The listing builds one solid part. Answer for the finished solid, in the listing's coordinates (mm). Face numbers are marked on the shaded views. A direction names the side the tool comes from. Round coordinates to 2 decimals unless told otherwise and drop trailing zeros. Write each loop counter-clockwise with the first axis right and the second up, starting at its lowest first coordinate (ties: lowest second). Pieces come first, ordered by that corner, then holes. Notation, with made-up numbers: (-21, -11) -> (-14, -11) arc R19 cw to (-14, -5) -> close; hole circle Ø3 at (38.25, 50.5). An arc over 180 degrees is marked (long way). Write each question's results on one line, items separated by ' | '. Start each with the question number.
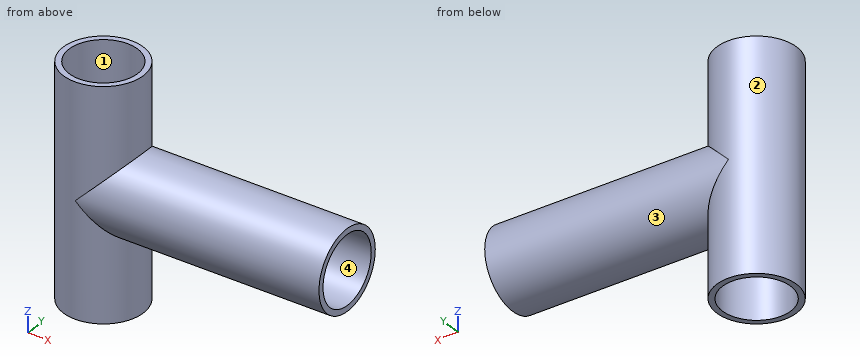
```python
from build123d import *

# Parameters (mm, degrees)
F0_R     = 17.5
F1_DEPTH = 100
F3_R     = 17.5
F4_DEPTH = 107.5
F5_R     = 15
F7_DEPTH = 95
F6_R     = 15
F8_DEPTH = 100


with BuildPart() as f1:
    # F0 (on Top) → F1 (new body)
    with BuildSketch(Plane.XY):
        Circle(F0_R)
    extrude(amount=F1_DEPTH)

    # F3 (on offset) → F4 (join)
    with BuildSketch(Plane.YZ.offset(107.5)):
        with Locations((0, 50)):
            Circle(F3_R)
    extrude(amount=-F4_DEPTH)

    # F5 (on face) → F7 (cut)
    with BuildSketch(Plane.YZ.offset(107.5)):
        with Locations((0, 50)):
            Circle(F5_R)
    extrude(amount=-F7_DEPTH, mode=Mode.SUBTRACT)

    # F6 (on face) → F8 (cut, through all)
    with BuildSketch(Plane.XY.offset(100)):
        Circle(F6_R)
    extrude(amount=-F8_DEPTH, mode=Mode.SUBTRACT)


solid = f1.part
```
Q1. The part is cut by section C-C, the plane z = 72. Write down the section's boundary in (x, y).
Q2. The part is cut by section D-D, the plane z = 50. Write down the section's boundary in (x, y).
Q3. Find the intervals of material crossed by line 1 (Z direction, x = 60, y = 0); line 2 (Y direction, x = 56, z = 50); line 3 (X direction, y = -10, z = 87), in increasing order.
Q4. Determine the mould class of the marked faces 3 and 4 for opening direction Y: pulls with the +Y half, pulls with the -Y half, needs draft (parallel to the pull), parting line crosses it, or undercut.
Q5. Each of these flat-tipped pins is pushed along its axis until it touches: pin 1 (1 mm diameter, centred on x = 89, y = 11.5, fed in from +Z); pin 2 (5.5 mm diameter, centred on y = 10.5, z = 49.5, fed in from +X); pin 3 (2 mm diameter, centred on y = 10, z = 18, fed in from -X). Where does it stop, or does it pass through?
Q6. The part is cut by section A-A, the plane y = 0. Write down the section's boundary in (x, z), then the cut area to 3 significant figures.
Q7. The part is cut by section B-B, the plane x = -8. Write down the section's boundary in (y, z).
Q8. For the marked faces 1 and 2, determine the directions among +Z, -Z, +X, -X, +Y, -Y from which every point of the face is accessible in a straight line to the end or side of a thin tool.
Answers follow:
1) outline: circle Ø35 at (0, 0); hole circle Ø30 at (0, 0)
2) outline: (0, -17.5) -> (107.5, -17.5) -> (107.5, -15) -> (12.5, -15) -> (12.5, -8.29) arc R15 cw (long way) to (12.5, 8.29) -> (12.5, 15) -> (107.5, 15) -> (107.5, 17.5) -> (0, 17.5) arc R17.5 ccw to start
3) line 1: 32.5 to 35, 65 to 67.5 | line 2: -17.5 to -15, 15 to 17.5 | line 3: -14.36 to -11.18, 11.18 to 14.36
4) face 3: parting line crosses it | face 4: undercut
5) pin 1: z = 63.61 | pin 2: x = 12.5 | pin 3: x = -15.01
6) outline: (-17.5, 0) -> (-15, 0) -> (-15, 100) -> (-17.5, 100) -> close; (15, 0) -> (17.5, 0) -> (17.5, 32.5) -> (107.5, 32.5) -> (107.5, 35) -> (15, 35) -> close; (15, 65) -> (107.5, 65) -> (107.5, 67.5) -> (17.5, 67.5) -> (17.5, 100) -> (15, 100) -> close | area: 875 mm^2
7) outline: (-15.56, 0) -> (-12.69, 0) -> (-12.69, 100) -> (-15.56, 100) -> close; (12.69, 0) -> (15.56, 0) -> (15.56, 100) -> (12.69, 100) -> close
8) face 1: +Z, -Z | face 2: none
